Geometry check sheet. Reference: the model listing, model coordinates, mm. A direction names the side the tool comes from. Round coordinates to 2 decimals unless told otherwise and drop trailing zeros. Loops run counter-clockwise (first coordinate to the right, second up) from the corner with the lowest first, then second, coordinate; pieces in that order, holes last. Notation, with made-up numbers: (30, -38.75) -> (34, -38.75) arc R19 ccw to (34, -25.75) -> close; hole circle Ø11 at (58, -5.5). An arc over 180 degrees is marked (long way). Use one line per item in the form item = value.
from build123d import *

# Parameters (mm, degrees)
F1_DEPTH  = 250
F2_R      = 7
F3_DEPTH  = 30
F4_DEPTH  = 30
F6_DEPTH  = 20
F8_DEPTH  = 20
F10_DEPTH = 30
F11_DEPTH = 30
F13_D     = 15
F13_DEPTH = 400
F13_TIP   = 4.5064546427
F15_D     = 5
F15_DEPTH = 10
F15_TIP   = 1.5021515476


with BuildPart() as f1:
    # F0 (on Front) → F1 (new body)
    with BuildSketch(Plane.XZ):
        with BuildLine():
            Line((0, 231.25), (0, 250))
            ThreePointArc((0, 250), (-176.7766952966, 176.7766952966), (-250, 0))
            Line((-250, 0), (-231.25, 0))
            ThreePointArc((-231.25, 0), (-163.5184431494, 163.5184431494), (0, 231.25))
        make_face()
    extrude(amount=F1_DEPTH)

    # F2 (on face) → F3 (join)
    with BuildSketch(Plane.YZ):
        with Locations((-208.4, 240.625)):
            Circle(F2_R)
        with Locations((-125, 240.625)):
            Circle(F2_R)
        with Locations((-41.6, 240.625)):
            Circle(F2_R)
    extrude(amount=F3_DEPTH)

    # F2 (on face) → F4 (cut)
    with BuildSketch(Plane.YZ):
        with Locations((-166.8, 240.625)):
            Circle(F2_R)
        with Locations((-83.2, 240.625)):
            Circle(F2_R)
    extrude(amount=-F4_DEPTH, mode=Mode.SUBTRACT)

    # F5 (on face) → F6 (join)
    with BuildSketch(Plane.XZ.offset(250)):
        with BuildLine():
            ThreePointArc((-211.25, 0), (-149.3763075257, 149.3763075257), (0, 211.25))
            Line((0, 211.25), (0, 231.25))
            ThreePointArc((0, 231.25), (-163.5184431494, 163.5184431494), (-231.25, 0))
            Line((-231.25, 0), (-211.25, 0))
        make_face()
    extrude(amount=-F6_DEPTH)

    # F7 (on face) → F8 (join)
    with BuildSketch(Plane(origin=(0, 0, 0), x_dir=(-1, 0, 0), z_dir=(0, 1, 0))):
        with BuildLine():
            ThreePointArc((0, 211.25), (149.3763075257, 149.3763075257), (211.25, 0))
            Line((211.25, 0), (231.25, 0))
            ThreePointArc((231.25, 0), (163.5184431494, 163.5184431494), (0, 231.25))
            Line((0, 231.25), (0, 211.25))
        make_face()
    extrude(amount=-F8_DEPTH)

    # F9 (on face) → F10 (join)
    with BuildSketch(Plane(origin=(0, 0, 0), x_dir=(1, 0, 0), z_dir=(0, 0, -1))):
        with BuildLine():
            Line((-240.625, 166.8), (-233.625, 166.8))
            ThreePointArc((-233.625, 166.8), (-235.6752525317, 171.7497474683), (-240.625, 173.8))
            Line((-240.625, 173.8), (-240.625, 166.8))
        make_face()
        with BuildLine():
            ThreePointArc((-240.625, 159.8), (-235.6752525317, 161.8502525317), (-233.625, 166.8))
            Line((-233.625, 166.8), (-240.625, 166.8))
            Line((-240.625, 166.8), (-240.625, 159.8))
        make_face()
        with BuildLine():
            Line((-240.625, 166.8), (-247.625, 166.8))
            ThreePointArc((-247.625, 166.8), (-245.5747474683, 161.8502525317), (-240.625, 159.8))
            Line((-240.625, 159.8), (-240.625, 166.8))
        make_face()
        with BuildLine():
            ThreePointArc((-240.625, 173.8), (-245.5747474683, 171.7497474683), (-247.625, 166.8))
            Line((-247.625, 166.8), (-240.625, 166.8))
            Line((-240.625, 166.8), (-240.625, 173.8))
        make_face()
        with BuildLine():
            Line((-240.625, 90.2), (-240.625, 83.2))
            Line((-240.625, 83.2), (-233.625, 83.2))
            ThreePointArc((-233.625, 83.2), (-235.6752525317, 88.1497474683), (-240.625, 90.2))
        make_face()
        with BuildLine():
            Line((-240.625, 83.2), (-240.625, 76.2))
            ThreePointArc((-240.625, 76.2), (-235.6752525317, 78.2502525317), (-233.625, 83.2))
            Line((-233.625, 83.2), (-240.625, 83.2))
        make_face()
        with BuildLine():
            Line((-247.625, 83.2), (-240.625, 83.2))
            Line((-240.625, 83.2), (-240.625, 90.2))
            ThreePointArc((-240.625, 90.2), (-245.5747474683, 88.1497474683), (-247.625, 83.2))
        make_face()
        with BuildLine():
            ThreePointArc((-247.625, 83.2), (-245.5747474683, 78.2502525317), (-240.625, 76.2))
            Line((-240.625, 76.2), (-240.625, 83.2))
            Line((-240.625, 83.2), (-247.625, 83.2))
        make_face()
    extrude(amount=F10_DEPTH)

    # F9 (on face) → F11 (cut)
    with BuildSketch(Plane(origin=(0, 0, 0), x_dir=(1, 0, 0), z_dir=(0, 0, -1))):
        with BuildLine():
            ThreePointArc((-240.625, 215.4), (-245.5747474683, 213.3497474683), (-247.625, 208.4))
            Line((-247.625, 208.4), (-240.625, 208.4))
            Line((-240.625, 208.4), (-240.625, 215.4))
        make_face()
        with BuildLine():
            Line((-240.625, 208.4), (-233.625, 208.4))
            ThreePointArc((-233.625, 208.4), (-235.6752525317, 213.3497474683), (-240.625, 215.4))
            Line((-240.625, 215.4), (-240.625, 208.4))
        make_face()
        with BuildLine():
            ThreePointArc((-240.625, 201.4), (-235.6752525317, 203.4502525317), (-233.625, 208.4))
            Line((-233.625, 208.4), (-240.625, 208.4))
            Line((-240.625, 208.4), (-240.625, 201.4))
        make_face()
        with BuildLine():
            Line((-240.625, 125), (-233.625, 125))
            ThreePointArc((-233.625, 125), (-235.6752525317, 129.9497474683), (-240.625, 132))
            Line((-240.625, 132), (-240.625, 125))
        make_face()
        with BuildLine():
            Line((-240.625, 125), (-247.625, 125))
            ThreePointArc((-247.625, 125), (-245.5747474683, 120.0502525317), (-240.625, 118))
            Line((-240.625, 118), (-240.625, 125))
        make_face()
        with BuildLine():
            ThreePointArc((-240.625, 118), (-235.6752525317, 120.0502525317), (-233.625, 125))
            Line((-233.625, 125), (-240.625, 125))
            Line((-240.625, 125), (-240.625, 118))
        make_face()
        with BuildLine():
            ThreePointArc((-240.625, 132), (-245.5747474683, 129.9497474683), (-247.625, 125))
            Line((-247.625, 125), (-240.625, 125))
            Line((-240.625, 125), (-240.625, 132))
        make_face()
        with BuildLine():
            Line((-240.625, 48.6), (-240.625, 41.6))
            Line((-240.625, 41.6), (-233.625, 41.6))
            ThreePointArc((-233.625, 41.6), (-235.6752525317, 46.5497474683), (-240.625, 48.6))
        make_face()
        with BuildLine():
            Line((-233.625, 41.6), (-240.625, 41.6))
            Line((-240.625, 41.6), (-240.625, 34.6))
            ThreePointArc((-240.625, 34.6), (-235.6752525317, 36.6502525317), (-233.625, 41.6))
        make_face()
        with BuildLine():
            Line((-247.625, 41.6), (-240.625, 41.6))
            Line((-240.625, 41.6), (-240.625, 48.6))
            ThreePointArc((-240.625, 48.6), (-245.5747474683, 46.5497474683), (-247.625, 41.6))
        make_face()
        with BuildLine():
            Line((-240.625, 34.6), (-240.625, 41.6))
            Line((-240.625, 41.6), (-247.625, 41.6))
            ThreePointArc((-247.625, 41.6), (-245.5747474683, 36.6502525317), (-240.625, 34.6))
        make_face()
        with BuildLine():
            Line((-240.625, 208.4), (-247.625, 208.4))
            ThreePointArc((-247.625, 208.4), (-245.5747474683, 203.4502525317), (-240.625, 201.4))
            Line((-240.625, 201.4), (-240.625, 208.4))
        make_face()
    extrude(amount=-F11_DEPTH, mode=Mode.SUBTRACT)

    # F13
    with Locations(Plane(origin=(0, 0, 0), x_dir=(-1, 0, 0), z_dir=(0, 1, 0))):
        with Locations((60.2965652341, 225.0298449755), (116.4840191922, 201.7562395108), (164.7332797414, 164.7332797414), (201.7562395108, 116.4840191922), (225.0298449755, 60.2965652341)):
            Hole(F13_D / 2, depth=F13_DEPTH)
            with Locations((0, 0, -(F13_DEPTH + F13_TIP / 2))):  # 118° drill point
                Cone(0, F13_D / 2, F13_TIP, mode=Mode.SUBTRACT)

    # F15 (one way)
    with BuildSketch(Plane.XZ.offset(20)):
        with Locations((-198.3330953711, 88.4955437344), (-172.1848046199, 134.3289181376), (-130.2505871514, 177.6727710928), (-79.6826335432, 207.8403590443)):
            Circle(F15_D / 2)
    extrude(amount=-F15_DEPTH, mode=Mode.SUBTRACT)
    with Locations(Plane.XZ.offset(20)):
        with Locations((-198.3330953711, 88.4955437344), (-172.1848046199, 134.3289181376), (-130.2505871514, 177.6727710928), (-79.6826335432, 207.8403590443)):
            with Locations((0, 0, -(F15_DEPTH + F15_TIP / 2))):  # 118° drill point
                Cone(0, F15_D / 2, F15_TIP, mode=Mode.SUBTRACT)


solid = f1.part
1. Section check B-B (z = 143.5). Record the boundary of the cut face in (x, y).
Return value:
outline = (-204.71, -250) -> (-155.03, -250) -> (-155.03, -230) -> (-181.34, -230) -> (-181.34, -20) -> (-155.03, -20) -> (-155.03, 0) -> (-204.71, 0) -> close
2. Section check A-A (y = -103). Record the boundary of the cut face in (x, z).
Return value:
outline = (-250, 0) -> (-231.25, 0) arc R231.25 cw to (-225.14, 52.8) arc R7.5 cw (long way) to (-221.38, 66.85) arc R231.25 cw to (-203.81, 109.27) arc R7.5 cw (long way) to (-196.53, 121.87) arc R231.25 cw to (-168.58, 158.29) arc R7.5 cw (long way) to (-158.29, 168.58) arc R231.25 cw to (-121.87, 196.53) arc R7.5 cw (long way) to (-109.27, 203.81) arc R231.25 cw to (-66.85, 221.38) arc R7.5 cw (long way) to (-52.8, 225.14) arc R231.25 cw to (0, 231.25) -> (0, 250) arc R250 ccw to start
3. Tool access check on faces 4 (the flat face through (30, -125, 241)), 5 (the flat face through (-149, -20, 150)), 6 (the flat face through (-30, -83, 241)). Record the directions out of +Z, -Z, +X, -X, +Y, -Y that give a thin tool (end or side, any length) a straight path to the whole face; none if there is none.
Return value:
face_4 = +Z, -Z, +X, +Y, -Y
face_5 = -Z, +X
face_6 = +X
4. Gauge pin test, flat ends, axial feed: pin 1 (4 mm diameter, centred on y = -160.5, z = 19, fed in from +X); pin 2 (5 mm diameter, centred on x = -185.5, y = -35, fed in from +Z); pin 3 (11.5 mm diameter, centred on y = -93.5, z = 228.5, fed in from +X); pin 4 (11.5 mm diameter, centred on x = -228.5, y = -85.5, fed in from -Z). Record the tip position at first contact, or that the pin passes through.
Return value:
pin_1 = -230.29
pin_2 = 170.33
pin_3 = 0
pin_4 = -30
5. Section check C-C (x = -136.5). Record the boundary of the cut face in (y, z).
Return value:
outline = (-250, 161.23) -> (-230, 161.23) -> (-230, 186.67) -> (-20, 186.67) -> (-20, 161.23) -> (0, 161.23) -> (0, 209.45) -> (-250, 209.45) -> close
6. Material ranges on line 1 along Y through (x, z) = (-238, 13); line 2 along X through (y, z) = (-69, 5); line 3 along X through (y, z) = (-23, 116), recorded low to high.
Return value:
line_1 = -250 to -214.89, -201.91 to -131.49, -118.51 to -48.09, -35.11 to 0
line_2 = -249.95 to -231.2
line_3 = -221.46 to -209.24
7. Mould release check, pull along X, two halves, no side actions. Record for faces 1 (the flat face through (-241, -208, 30)), 2 (the cylindrical face through (-183.66, -123.53, 140.52)), 3 (the cylindrical face through (14.79, -130.555, 236.366)): released by +X, released by -X, zero draft, split by the parting line, or undercut.
Return value:
face_1 = undercut
face_2 = released by +X
face_3 = zero draft
